Input: part model. Units: mm. Frame: model coordinates. A direction names the side the tool comes from. Round coordinates to 2 decimals unless told otherwise and drop trailing zeros. Loops run counter-clockwise (first coordinate to the right, second up) from the corner with the lowest first, then second, coordinate; pieces in that order, holes last. Notation, with made-up numbers: (70.5, 75.25) - (102.5, 75.25) arc R8 cw to (102.5, 87.25) - close; hole circle Ø10 at (-17, 35). An arc over 180 degrees is marked (long way). Use CSV: the item, a comma, the result in double quotes. Start each with the question number.
1. Pull-direction query (Z, two-part tool) for faces 1 (the flat face through (65, 10, -62.1)), 2 (the flat face through (0, 20, 60)), 3 (the cylindrical face through (-49, 9.9, -58.7)); classes: +Z half, -Z half, draft (parallel to the pull), parting line (faces both ways), or undercut.
2. Material intervals for probe 1 along X at (y, z) = (18.25, -3); probe 2 along Z at (x, y) = (39, 12.5); probe 3 along X at (y, z) = (6.25, 54.5), sorted ascending. Write a range as from..to.
3. Cut plane B-B (y = 2). Return loops of the section in (x, z), and give its area (3 significant figures).
4. Cut plane C-C (x = -24). Return loops of the section in (y, z), and give its area (3 significant figures).
5. Pin query (flat end, axial travel): P1, Ø1.6, axis at y = 10, z = -60.5, coming from the +X side. Return the tip coordinate at first contact, or that it passes through.
6. Cut plane A-A (z = 35.5). Return loops of the section in (x, y).
7. Access query for faces 4 (the flat face through (-1, 10, 55.1)), 5 (the flat face through (80.2, 10, 1)). Directions: +Z, -Z, +X, -X, +Y, -Y. A direction counts if a zero-diameter tool reaches every point of the face in a straight line with its end or side. Return the directions, or none.
```python
from build123d import *

# Parameters (mm, degrees)
ESBO_O1_W                    = 160.4
ESBO_O1_H                    = 124.2
ESBO_O1_W_2                  = 146.4
ESBO_O1_H_2                  = 110.2
PAREDES_DEPTH                = 20
CHANFROS_INTERNO_FRENTE_SIZE = 5
FILETE1_R                    = 3
FILETE2_R                    = 3
ESBO_O2_W                    = 98
ESBO_O2_H                    = 30
CORTE_EXTRUS_O1_DEPTH        = 20
FILETE3_RADIUS               = 3.5
FILETE3_LENGTH               = 20
FILETE4_RADIUS               = 3.5
FILETE4_LENGTH               = 20
FILETE5_R                    = 3
FILETE6_R                    = 3
CHANFRO2_SIZE                = 3


with BuildPart() as part:
    # Esboço1 → Paredes (new body)
    with BuildSketch(Plane(origin=(0, 0, 0), x_dir=(1, 0, 0), z_dir=(0, 1, 0))):
        Rectangle(ESBO_O1_W, ESBO_O1_H)
        Rectangle(ESBO_O1_W_2, ESBO_O1_H_2, mode=Mode.SUBTRACT)
    extrude(amount=PAREDES_DEPTH)

    # Chanfros Interno Frente
    chanfros_interno_frente_edges = [part.edges().sort_by_distance(p)[0] for p in [
        (73.2, 10, 55.1),
        (-73.2, 10, 55.1),
    ]]
    chamfer(chanfros_interno_frente_edges, length=CHANFROS_INTERNO_FRENTE_SIZE)

    # Filete1
    filete1_edges = [part.edges().sort_by_distance(p)[0] for p in [
        (-80.2, 10, 62.1),
    ]]
    fillet(filete1_edges, radius=FILETE1_R)

    # Filete2
    filete2_edges = [part.edges().sort_by_distance(p)[0] for p in [
        (80.2, 10, 62.1),
    ]]
    fillet(filete2_edges, radius=FILETE2_R)

    # Esboço2 → Corte-extrusão1 (cut)
    with BuildSketch(Plane(origin=(0, 0, -62.1), x_dir=(-1, 0, 0), z_dir=(0, 0, -1))):
        with Locations((0, 10)):
            Rectangle(ESBO_O2_W, ESBO_O2_H)
        with BuildLine():
            Line((58.5, 11), (58.5, 9))
            ThreePointArc((58.5, 9), (58.939339828, 7.939339828), (60, 7.5))
            Line((60, 7.5), (62, 7.5))
            ThreePointArc((62, 7.5), (63.060660172, 7.939339828), (63.5, 9))
            Line((63.5, 9), (63.5, 11))
            ThreePointArc((63.5, 11), (63.060660172, 12.060660172), (62, 12.5))
            Line((62, 12.5), (60, 12.5))
            ThreePointArc((60, 12.5), (58.939339828, 12.060660172), (58.5, 11))
        make_face()
        with BuildLine():
            Line((-62, 12.5), (-60, 12.5))
            ThreePointArc((-60, 12.5), (-58.939339828, 12.060660172), (-58.5, 11))
            Line((-58.5, 11), (-58.5, 9))
            ThreePointArc((-58.5, 9), (-58.939339828, 7.939339828), (-60, 7.5))
            Line((-60, 7.5), (-62, 7.5))
            ThreePointArc((-62, 7.5), (-63.060660172, 7.939339828), (-63.5, 9))
            Line((-63.5, 9), (-63.5, 11))
            ThreePointArc((-63.5, 11), (-63.060660172, 12.060660172), (-62, 12.5))
        make_face()
    extrude(amount=-CORTE_EXTRUS_O1_DEPTH, mode=Mode.SUBTRACT)

    # Filete3: full round fillet: the end face becomes a half cylinder, R = half its width
    filete3_face = Plane((49, 10, -58.6), x_dir=(0, 1, 0), z_dir=(-1, 0, 0))  # on the end face: x along it, z out of the body
    filete3_slab = filete3_face.offset(-FILETE3_RADIUS / 2) * Box(FILETE3_LENGTH, 2 * FILETE3_RADIUS, FILETE3_RADIUS, mode=Mode.PRIVATE)  # the body's end, R deep
    filete3_round = Plane((52.5, 10, -58.6), x_dir=(-1, 0, 0), z_dir=(0, 1, 0)) * Cylinder(FILETE3_RADIUS, FILETE3_LENGTH, mode=Mode.PRIVATE)  # its axis R under the face
    add(filete3_slab - filete3_round, mode=Mode.SUBTRACT)

    # Filete4: full round fillet: the end face becomes a half cylinder, R = half its width
    filete4_face = Plane((-49, 10, -58.6), x_dir=(0, -1, 0), z_dir=(1, 0, 0))  # on the end face: x along it, z out of the body
    filete4_slab = filete4_face.offset(-FILETE4_RADIUS / 2) * Box(FILETE4_LENGTH, 2 * FILETE4_RADIUS, FILETE4_RADIUS, mode=Mode.PRIVATE)  # the body's end, R deep
    filete4_round = Plane((-52.5, 10, -58.6), x_dir=(1, 0, 0), z_dir=(0, -1, 0)) * Cylinder(FILETE4_RADIUS, FILETE4_LENGTH, mode=Mode.PRIVATE)  # its axis R under the face
    add(filete4_slab - filete4_round, mode=Mode.SUBTRACT)

    # Filete5
    filete5_edges = [part.edges().sort_by_distance(p)[0] for p in [
        (-80.2, 10, -62.1),
    ]]
    fillet(filete5_edges, radius=FILETE5_R)

    # Filete6
    filete6_edges = [part.edges().sort_by_distance(p)[0] for p in [
        (80.2, 10, -62.1),
    ]]
    fillet(filete6_edges, radius=FILETE6_R)

    # Chanfro2
    chanfro2_edges = [part.edges().sort_by_distance(p)[0] for p in [
        (73.2, 10, -55.1),
        (-73.2, 10, -55.1),
    ]]
    chamfer(chanfro2_edges, length=CHANFRO2_SIZE)


solid = part.part
```
Established:
1,face 1,"-Z half"
1,face 2,"draft"
1,face 3,"undercut"
2,probe 1,"x = -80.2..-73.2, 73.2..80.2"
2,probe 2,"z = 55.1..62.1"
2,probe 3,"x = -80.2..-68.8, 68.8..80.2"
3,outline,"(-80.2, -59.1) arc R3 ccw to (-77.2, -62.1) - (-52.5, -62.1) arc R3.5 ccw to (-52.5, -55.1) - (-70.2, -55.1) - (-73.2, -52.1) - (-73.2, 50.1) - (-68.2, 55.1) - (68.2, 55.1) - (73.2, 50.1) - (73.2, -52.1) - (70.2, -55.1) - (52.5, -55.1) arc R3.5 ccw to (52.5, -62.1) - (77.2, -62.1) arc R3 ccw to (80.2, -59.1) - (80.2, 59.1) arc R3 ccw to (77.2, 62.1) - (-77.2, 62.1) arc R3 ccw to (-80.2, 59.1) - close"
3,area,"3,120 mm2"
4,outline,"(0, 55.1) - (20, 55.1) - (20, 62.1) - (0, 62.1) - close"
4,area,"140 mm2"
5,P1,"stops at x = 80.14"
6,outline,"(-80.2, 0) - (-73.2, 0) - (-73.2, 20) - (-80.2, 20) - close; (73.2, 0) - (80.2, 0) - (80.2, 20) - (73.2, 20) - close"
7,face 4,"+Y, -Y"
7,face 5,"+Z, -Z, +X, +Y, -Y"
